Source: CAD feature listing. Evaluate the final solid. Frame: model axes, mm. Give positions to 0.01 mm unless a question says otherwise; leave off trailing zeros. Loops run counter-clockwise (first coordinate to the right, second up) from the corner with the lowest first, then second, coordinate; pieces in that order, holes last.
from build123d import *

# Parameters (mm, degrees)
BOSS_EXTRUDE1_DEPTH    = 1.5875
F_10_CLEARANCE_HOLE1_D = 5.1054


with BuildPart() as part:
    # Sketch3 → Boss-Extrude1 (new body)
    with BuildSketch(Plane(origin=(0, 0, 0), x_dir=(1, 0, 0), z_dir=(0, 1, 0))):
        Polygon((-96.156504736, -35.371535332), (-96.156504736, 240.853464665), (-70.756504733, 266.253464668), (110.218495843, 266.253464668), (135.618495843, 240.853464668), (135.618495843, -3.621535332), (-70.756504661, -3.621535332), (-70.756504661, -35.371535332), align=None)
    extrude(amount=BOSS_EXTRUDE1_DEPTH)

    # #10 Clearance Hole1 (through all)
    with Locations(Plane(origin=(0, 1.5875, 0), x_dir=(1, 0, 0), z_dir=(0, 1, 0))):
        with Locations((-83.456504705, -25.846534826), (-83.456504732, 202.753465682), (-83.456504732, 228.153465682), (-70.756504732, 253.553465682), (122.918495843, 202.753464668), (122.918495843, 228.153464668), (110.218495843, 253.553464668)):
            Hole(F_10_CLEARANCE_HOLE1_D / 2)


solid = part.part
1) Cut plane B-B (x = -55). Return loops of the section in (y, z), and give its area (3 significant figures).
Checks:
outline: (0, -266.25) - (1.59, -266.25) - (1.59, 3.62) - (0, 3.62) - close
area: 428 mm2
2) Cut plane C-C (z = 12). Return loops of the section in (x, y), and give its area (3 significant figures).
Checks:
outline: (-96.16, 0) - (-70.76, 0) - (-70.76, 1.59) - (-96.16, 1.59) - close
area: 40.3 mm2
3) Cut plane A-A (y = 0.3). Return loops of the section in (x, z).
Checks:
outline: (-96.16, -240.85) - (-70.76, -266.25) - (110.22, -266.25) - (135.62, -240.85) - (135.62, 3.62) - (-70.76, 3.62) - (-70.76, 35.37) - (-96.16, 35.37) - close; hole circle Ø5.11 at (-83.46, -228.15); hole circle Ø5.11 at (-83.46, -202.75); hole circle Ø5.11 at (-83.46, 25.85); hole circle Ø5.11 at (-70.76, -253.55); hole circle Ø5.11 at (110.22, -253.55); hole circle Ø5.11 at (122.92, -228.15); hole circle Ø5.11 at (122.92, -202.75)
4) Contact query for flat-ended pins moving along their axis: P1, Ø3, axis at x = -83.46, z = -202.75, coming from the -Y side; P2, Ø6.5, axis at x = 110.22, z = -253.55, coming from the +Y side; P3, Ø0.5, axis at y = 1, z = 24.5, coming from the +X side. Output: stop coordinate, or through.
Checks:
P1: passes through
P2: stops at y = 1.59
P3: stops at x = -70.76
5) Ray query, probe 1 along Z at (x, y) = (110, 1.45); probe 2 along Z at (x, y) = (-1, 1); probe 3 along X at (y, z) = (1.4, 19). Return the intervals inside material, ascending.
Checks:
probe 1: z = -266.25 to -256.1, -251.01 to 3.62
probe 2: z = -266.25 to 3.62
probe 3: x = -96.16 to -70.76
